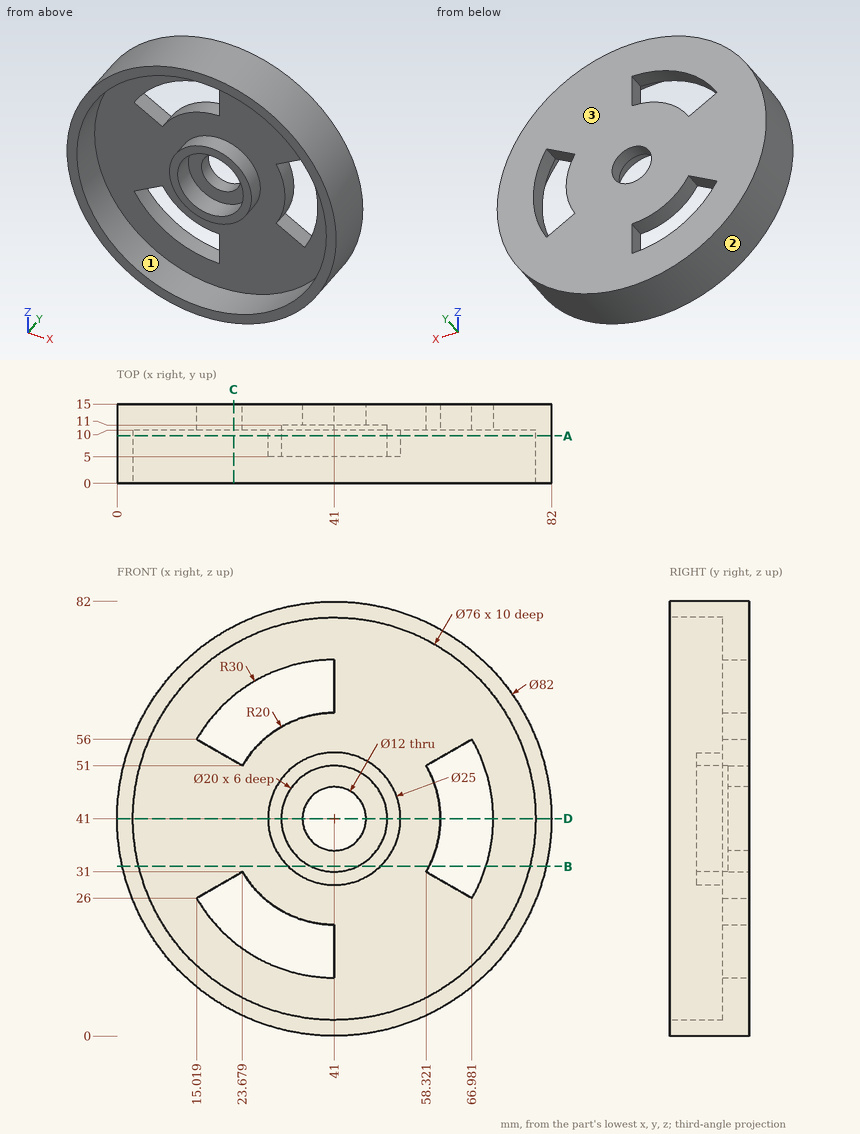
Answer from the drawing. Dimensions are ordinates in mm from the lowest x, y and z of the part. Give positions to 0.01 mm unless a question says otherwise; leave off trailing zeros. Loops run counter-clockwise (first coordinate to the right, second up) from the corner with the lowest first, then second, coordinate; pieces in that order, holes last. Notation, with made-up numbers: (55, 41) - (104, 41) arc R16 ccw to (104, 58) - close; hole circle Ø2 at (2, -11.75). An arc over 180 degrees is marked (long way). Write each question's results on one line, items separated by ' | '.
1. Flat-ended cylindrical pins translate along their axes: P1, Ø16, axis at x = 41, z = 41, coming from the -Y side; P2, Ø4, axis at x = 28.5, y = 11, coming from the -Z side; P3, Ø1, axis at x = 9, y = 5.5, coming from the -Z side (1 decimal). Find the tip coordinate at first contact, or state that the pin passes through.
Resolved:
P1: stops at y = 11 | P2: stops at z = 1.37 | P3: stops at z = 14.8
2. Find section D-D, the plane z = 41. Write down the section's boundary in (x, y).
Resolved:
outline: (0, 0) - (3, 0) - (3, 10) - (28.5, 10) - (28.5, 5) - (31, 5) - (31, 11) - (35, 11) - (35, 15) - (0, 15) - close; (47, 11) - (51, 11) - (51, 5) - (53.5, 5) - (53.5, 10) - (61, 10) - (61, 15) - (47, 15) - close; (71, 10) - (79, 10) - (79, 0) - (82, 0) - (82, 15) - (71, 15) - close
3. Find section C-C, the plane x = 22. Write down the section's boundary in (y, z), then the cut area to 3 significant figures.
Resolved:
outline: (0, 4.67) - (15, 4.67) - (15, 17.78) - (10, 17.78) - (10, 8.09) - (0, 8.09) - close; (0, 73.91) - (10, 73.91) - (10, 64.22) - (15, 64.22) - (15, 77.33) - (0, 77.33) - close; (10, 30.03) - (15, 30.03) - (15, 51.97) - (10, 51.97) - close | area: 309 mm^2
4. Find section A-A, the plane y = 9. Write down the section's boundary in (x, z).
Resolved:
outline: circle Ø82 at (41, 41); circle Ø25 at (41, 41); hole circle Ø76 at (41, 41); hole circle Ø20 at (41, 41)
5. Find section B-B, the plane z = 32. Write down the section's boundary in (x, y) (1 decimal).
Resolved:
outline: (1, 0) - (4.1, 0) - (4.1, 10) - (32.3, 10) - (32.3, 5) - (36.6, 5) - (36.6, 11) - (45.4, 11) - (45.4, 5) - (49.7, 5) - (49.7, 10) - (58.9, 10) - (58.9, 15) - (1, 15) - close; (69.6, 10) - (77.9, 10) - (77.9, 0) - (81, 0) - (81, 15) - (69.6, 15) - close
6. Consider probe 1 along Z at (x, y) = (41, 6.25); probe 2 along X at (y, z) = (3, 41); probe 3 along Z at (x, y) = (17, 14.25) (1 decimal). Determine where each line is inside the solid, lowest interval first. Write a range as from..to.
Resolved:
probe 1: z = 0..3, 28.5..31, 51..53.5, 79..82 | probe 2: x = 0..3, 79..82 | probe 3: z = 7.8..23, 27.1..54.9, 59..74.2
7. For a pull along X with two mould halves and no side action, classify the marked faces 1, 2 and 3 as +X half, -X half, draft (parallel to the pull), parting line (faces both ways), or undercut.
Resolved:
face 1: undercut | face 2: parting line | face 3: draft
